Model file for the job. Use its own axes, mm. Face numbers are marked on the shaded views. A direction names the side the tool comes from. Round coordinates to 2 decimals unless told otherwise and drop trailing zeros. Loops run counter-clockwise (first coordinate to the right, second up) from the corner with the lowest first, then second, coordinate; pieces in that order, holes last. Notation, with made-up numbers: M 43.5,50 L 102.5,50 A12 ccw 102.5,59 Z; hole C 52,-7 d1. An arc over 180 degrees is marked long. Use a Markdown table: item, result. Add a question column.
Q1. Probe line 1 (Z direction, x = -33, y = 18) (3 decimals); line 2 (Z direction, x = -33.85, y = 18) (3 decimals); line 3 (X direction, y = 7, z = 7). List the from-to ranges inside material, lowest first. Write a range as from..to.
Q2. Cut at C-C (x = -15.5). Give the cut face in (y, z) (3 decimals).
Q3. Tool access for the marked faces 1, 2, 3 and 4: list every direction of +Z, -Z, +X, -X, +Y, -Y with a clear straight run to the whole face (end or side of a thin tool).
Q4. Pin check, flat tips, straight feed: pin 1 (1.6 mm diameter, centred on x = -36.5, y = 18, fed in from +Z); pin 2 (2.5 mm diameter, centred on x = 5.5, y = 24, fed in from +Z) (3 decimals); pin 3 (6 mm diameter, centred on x = 27, z = -13, fed in from -Y); pin 4 (6 mm diameter, centred on x = -28, z = -6.5, fed in from +Y). Stop position of each tip, or through.
Q5. Cut at A-A (y = 0). Give the cut face in (x, z) (3 decimals).
Q6. Cut at B-B (x = -3). Give the cut face in (y, z) (3 decimals).
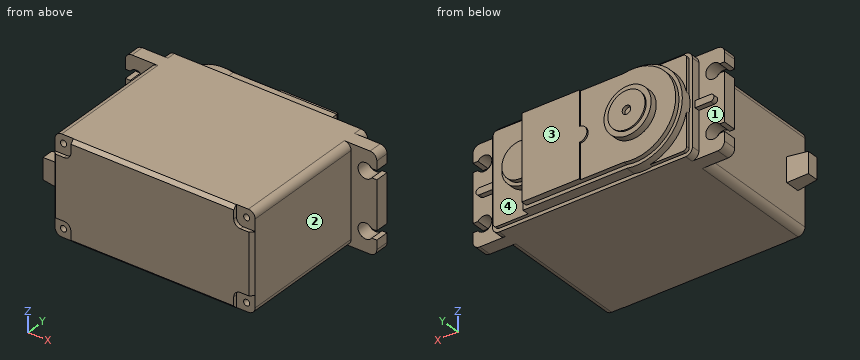
from build123d import *

# Parameters (mm, degrees)
CROQUIS1_W                      = 59.1
CROQUIS1_H                      = 28.85
SALIENTE_EXTRUIR1_DEPTH         = 22.65
CORTAR_EXTRUIR1_DEPTH           = 1.1
CHAFL_N1_SIZE                   = 1
REDONDEO1_R                     = 2
SALIENTE_EXTRUIR2_DEPTH         = 4
REDONDEO2_R                     = 2
SALIENTE_EXTRUIR3_DEPTH         = 1.5
SALIENTE_EXTRUIR4_DEPTH         = 1
SALIENTE_EXTRUIR5_DEPTH         = 3
SALIENTE_EXTRUIR6_DEPTH         = 1.3
CROQUIS8_R                      = 6.96
SALIENTE_EXTRUIR7_DEPTH         = 2
CROQUIS9_R                      = 5.485
SALIENTE_EXTRUIR8_DEPTH         = 0.44
CROQUIS10_R                     = 1.25
CORTAR_EXTRUIR2_DEPTH           = 1
TALADRO_DE_MARGEN_PARA_81_D     = 4.4958
TALADRO_DE_MARGEN_PARA_81_DEPTH = 4
SALIENTE_EXTRUIR9_DEPTH         = 0.5
CROQUIS17_W                     = 7.24
CROQUIS17_H                     = 4.41
CROQUIS18_W                     = 6.24
CROQUIS18_H                     = 3.41


with BuildPart() as part:
    # Croquis1 → Saliente-Extruir1 (new body, symmetric)
    with BuildSketch(Plane(origin=(0, 0, 0), x_dir=(1, 0, 0), z_dir=(0, 1, 0))):
        Rectangle(CROQUIS1_W, CROQUIS1_H)
    extrude(amount=SALIENTE_EXTRUIR1_DEPTH, both=True)

    # Croquis2 → Cortar-Extruir1 (cut)
    with BuildSketch(Plane.XZ.offset(22.65)):
        with BuildLine():
            Line((29.55, 14.425), (24.05, 14.425))
            Line((24.05, 14.425), (24.05, 10.925))
            ThreePointArc((24.05, 10.925), (24.635786438, 9.510786438), (26.05, 8.925))
            Line((26.05, 8.925), (29.55, 8.925))
            Line((29.55, 8.925), (29.55, 14.425))
        make_face()
        with BuildLine():
            Line((-29.55, 14.425), (-29.55, 8.925))
            Line((-29.55, 8.925), (-26.05, 8.925))
            ThreePointArc((-26.05, 8.925), (-24.635786438, 9.510786438), (-24.05, 10.925))
            Line((-24.05, 10.925), (-24.05, 14.425))
            Line((-24.05, 14.425), (-29.55, 14.425))
        make_face()
        with BuildLine():
            Line((24.05, -14.425), (24.05, -10.925))
            ThreePointArc((24.05, -10.925), (24.635786438, -9.510786438), (26.05, -8.925))
            Line((26.05, -8.925), (29.55, -8.925))
            Line((29.55, -8.925), (29.55, -14.425))
            Line((29.55, -14.425), (24.05, -14.425))
        make_face()
        with BuildLine():
            Line((-24.05, -14.425), (-24.05, -10.925))
            ThreePointArc((-24.05, -10.925), (-24.635786438, -9.510786438), (-26.05, -8.925))
            Line((-26.05, -8.925), (-29.55, -8.925))
            Line((-29.55, -8.925), (-29.55, -14.425))
            Line((-29.55, -14.425), (-24.05, -14.425))
        make_face()
    extrude(amount=-CORTAR_EXTRUIR1_DEPTH, mode=Mode.SUBTRACT)

    # Chaflán1
    chafl_n1_edges = [part.edges().sort_by_distance(p)[0] for p in [
        (29.55, -22.65, 0),
        (0, -22.65, 14.425),
        (0, -22.65, -14.425),
        (-29.55, -22.65, 0),
    ]]
    chamfer(chafl_n1_edges, length=CHAFL_N1_SIZE)

    # Redondeo1
    redondeo1_edges = [part.edges().sort_by_distance(p)[0] for p in [
        (29.55, 0.55, 14.425),
        (-29.55, 0.55, 14.425),
        (-29.55, 0.55, -14.425),
        (29.55, 0.55, -14.425),
    ]]
    fillet(redondeo1_edges, radius=REDONDEO1_R)

    # Croquis3 → Saliente-Extruir2 (add)
    with BuildSketch(Plane(origin=(0, 16.15, 0), x_dir=(1, 0, 0), z_dir=(0, 1, 0))):
        with BuildLine():
            Line((27.55, 14.425), (37.15, 14.425))
            Line((37.15, 14.425), (37.15, 9.725))
            Line((37.15, 9.725), (35.599971428, 9.725))
            Line((35.599971428, 9.725), (35.599971428, 7.125))
            Line((35.599971428, 7.125), (37.15, 7.125))
            Line((37.15, 7.125), (37.15, -7.125))
            Line((37.15, -7.125), (35.599971428, -7.125))
            Line((35.599971428, -7.125), (35.599971428, -9.725))
            Line((35.599971428, -9.725), (37.15, -9.725))
            Line((37.15, -9.725), (37.15, -14.425))
            Line((37.15, -14.425), (27.55, -14.425))
            ThreePointArc((27.55, -14.425), (28.964213562, -13.839213562), (29.55, -12.425))
            Line((29.55, -12.425), (29.55, 12.425))
            ThreePointArc((29.55, 12.425), (28.964213562, 13.839213562), (27.55, 14.425))
        make_face()
        with BuildLine():
            Line((-37.15, -9.725), (-37.15, -14.425))
            Line((-37.15, -14.425), (-27.55, -14.425))
            ThreePointArc((-27.55, -14.425), (-28.964213562, -13.839213562), (-29.55, -12.425))
            Line((-29.55, -12.425), (-29.55, 12.425))
            ThreePointArc((-29.55, 12.425), (-28.964213562, 13.839213562), (-27.55, 14.425))
            Line((-27.55, 14.425), (-37.15, 14.425))
            Line((-37.15, 14.425), (-37.15, 9.725))
            Line((-37.15, 9.725), (-35.599971428, 9.725))
            Line((-35.599971428, 9.725), (-35.599971428, 7.125))
            Line((-35.599971428, 7.125), (-37.15, 7.125))
            Line((-37.15, 7.125), (-37.15, -7.125))
            Line((-37.15, -7.125), (-35.599971428, -7.125))
            Line((-35.599971428, -7.125), (-35.599971428, -9.725))
            Line((-35.599971428, -9.725), (-37.15, -9.725))
        make_face()
    extrude(amount=SALIENTE_EXTRUIR2_DEPTH)

    # Redondeo2
    redondeo2_edges = [part.edges().sort_by_distance(p)[0] for p in [
        (37.15, 18.15, 14.425),
        (37.15, 18.15, -14.425),
        (-37.15, 18.15, 14.425),
        (-37.15, 18.15, -14.425),
    ]]
    fillet(redondeo2_edges, radius=REDONDEO2_R)

    # Croquis4 → Saliente-Extruir3 (add)
    with BuildSketch(Plane(origin=(0, 20.15, 0), x_dir=(1, 0, 0), z_dir=(0, 1, 0))):
        with BuildLine():
            Line((34.13221447, -1), (29.55, -1))
            Line((29.55, -1), (29.55, 1))
            Line((29.55, 1), (34.13221447, 1))
            ThreePointArc((34.13221447, 1), (35.13221447, 0), (34.13221447, -1))
        make_face()
        with BuildLine():
            Line((-29.55, -1), (-29.55, 1))
            Line((-29.55, 1), (-34.13221447, 1))
            ThreePointArc((-34.13221447, 1), (-35.13221447, 0), (-34.13221447, -1))
            Line((-34.13221447, -1), (-29.55, -1))
        make_face()
    extrude(amount=SALIENTE_EXTRUIR3_DEPTH)

    # Croquis5 → Saliente-Extruir4 (add)
    with BuildSketch(Plane(origin=(0, 22.65, 0), x_dir=(1, 0, 0), z_dir=(0, 1, 0))):
        with BuildLine():
            Line((-27.55, -13.425), (27.55, -13.425))
            ThreePointArc((27.55, -13.425), (28.257106781, -13.132106781), (28.55, -12.425))
            Line((28.55, -12.425), (28.55, 12.425))
            ThreePointArc((28.55, 12.425), (28.257106781, 13.132106781), (27.55, 13.425))
            Line((27.55, 13.425), (-27.55, 13.425))
            ThreePointArc((-27.55, 13.425), (-28.257106781, 13.132106781), (-28.55, 12.425))
            Line((-28.55, 12.425), (-28.55, -12.425))
            ThreePointArc((-28.55, -12.425), (-28.257106781, -13.132106781), (-27.55, -13.425))
        make_face()
    extrude(amount=SALIENTE_EXTRUIR4_DEPTH)

    # Croquis6 → Saliente-Extruir5 (add)
    with BuildSketch(Plane(origin=(0, 22.65, 0), x_dir=(1, 0, 0), z_dir=(0, 1, 0))):
        with BuildLine():
            Line((-12.39381436, 13.425), (18.25, 13.425))
            Line((18.25, 13.425), (18.25, 6.275))
            ThreePointArc((18.25, 6.275), (24.525, 0), (18.25, -6.275))
            Line((18.25, -6.275), (18.25, -13.425))
            Line((18.25, -13.425), (-12.39381436, -13.425))
            ThreePointArc((-12.39381436, -13.425), (-28.825, 0), (-12.39381436, 13.425))
        make_face()
    extrude(amount=SALIENTE_EXTRUIR5_DEPTH)

    # Croquis7 → Saliente-Extruir6 (add)
    with BuildSketch(Plane(origin=(0, 25.65, 0), x_dir=(1, 0, 0), z_dir=(0, 1, 0))):
        with BuildLine():
            Line((17.25, 5.179346001), (17.25, 12.425))
            Line((17.25, 12.425), (-12.496430998, 12.425))
            ThreePointArc((-12.496430998, 12.425), (-27.825, 0), (-12.496430998, -12.425))
            Line((-12.496430998, -12.425), (17.25, -12.425))
            Line((17.25, -12.425), (17.25, -5.179346001))
            ThreePointArc((17.25, -5.179346001), (23.525, 0), (17.25, 5.179346001))
        make_face()
    extrude(amount=SALIENTE_EXTRUIR6_DEPTH)

    # Croquis8 → Saliente-Extruir7 (add)
    with BuildSketch(Plane(origin=(0, 26.95, 0), x_dir=(1, 0, 0), z_dir=(0, 1, 0))):
        with Locations((-15.125, 0)):
            Circle(CROQUIS8_R)
    extrude(amount=SALIENTE_EXTRUIR7_DEPTH)

    # Croquis9 → Saliente-Extruir8 (add)
    with BuildSketch(Plane(origin=(0, 28.95, 0), x_dir=(1, 0, 0), z_dir=(0, 1, 0))):
        with Locations((-15.125, 0)):
            Circle(CROQUIS9_R)
    extrude(amount=SALIENTE_EXTRUIR8_DEPTH)

    # Croquis10 → Cortar-Extruir2 (cut)
    with BuildSketch(Plane(origin=(0, 29.39, 0), x_dir=(1, 0, 0), z_dir=(0, 1, 0))):
        with Locations((-15.125, 0)):
            Circle(CROQUIS10_R)
    extrude(amount=-CORTAR_EXTRUIR2_DEPTH, mode=Mode.SUBTRACT)

    # Croquis11 → Taladro de margen para M1.61 (revolve, cut)
    with BuildSketch(Plane(origin=(27.05, -21.55, -11.925), x_dir=(0, 0, -1), z_dir=(1, 0, 0))):
        Polygon((0, 0), (0, 5.540774557), (0.9, 5), (0.9, 0), align=None)
    taladro_de_margen_para_m1_61 = revolve(axis=Axis((27.05, -27.9, -11.925), (0, 1, 0)), mode=Mode.SUBTRACT)

    # Simetría1: Taladro de margen para M1.61 across plane
    add(taladro_de_margen_para_m1_61.mirror(Plane.XY), mode=Mode.SUBTRACT)

    # Simetría2: Taladro de margen para M1.61 across plane
    add(taladro_de_margen_para_m1_61.mirror(Plane(origin=(0, 0, 0), x_dir=(0, 0, 1), z_dir=(1, 0, 0))), mode=Mode.SUBTRACT)

    # Simetría2 copy 1 sketch → Simetría2 copy 1 (revolve, cut)
    with BuildSketch(Plane(origin=(-27.05, -21.55, 11.925), x_dir=(0, 0, 1), z_dir=(-1, 0, 0))):
        Polygon((0, 0), (0, 5.540774557), (0.9, 5), (0.9, 0), align=None)
    revolve(axis=Axis((-27.05, -27.9, 11.925), (0, 1, 0)), mode=Mode.SUBTRACT)

    # Taladro de margen para #81
    with Locations(Plane(origin=(0, 20.15, 0), x_dir=(1, 0, 0), z_dir=(0, 1, 0))):
        with Locations((33.85, 8.425), (33.85, -8.425), (-33.85, 8.425), (-33.85, -8.425)):
            Hole(TALADRO_DE_MARGEN_PARA_81_D / 2, depth=TALADRO_DE_MARGEN_PARA_81_DEPTH)

    # Croquis15 → Saliente-Extruir9 (add)
    with BuildSketch(Plane(origin=(0, 26.95, 0), x_dir=(1, 0, 0), z_dir=(0, 1, 0))):
        with BuildLine():
            Line((17.25, 12.425), (0.25, 12.425))
            Line((0.25, 12.425), (0.25, 2.23))
            ThreePointArc((0.25, 2.23), (-1.98, 0), (0.25, -2.23))
            Line((0.25, -2.23), (0.25, -12.425))
            Line((0.25, -12.425), (17.25, -12.425))
            Line((17.25, -12.425), (17.25, 12.425))
        make_face()
    extrude(amount=SALIENTE_EXTRUIR9_DEPTH)

    # Croquis17 → Recubrir1 section 0
    with BuildSketch(Plane.ZY.offset(29.55)):
        with Locations((0, -16.595)):
            Rectangle(CROQUIS17_W, CROQUIS17_H)
    # Croquis18 → Recubrir1 section 1
    with BuildSketch(Plane.ZY.offset(35.55)):
        with Locations((0, -16.595)):
            Rectangle(CROQUIS18_W, CROQUIS18_H)
    loft()


solid = part.part
Checked values:
| question | item | result |
|---|---|---|
| 1 | line 1 | z = -14.425..-10.506, -6.344..6.344, 10.506..14.425 |
| 1 | line 2 | z = -14.425..-10.673, -6.177..6.177, 10.673..14.425 |
| 1 | line 3 | x = -29.55..29.55 |
| 2 | outline | M -22.65,-13.425 L -21.65,-14.425 L 22.65,-14.425 L 22.65,-13.695 L 25.65,-13.695 L 25.65,-12.694 L 26.95,-12.694 L 26.95,-6.95 L 28.95,-6.95 L 28.95,-5.472 L 29.39,-5.472 L 29.39,-1.192 L 28.39,-1.192 L 28.39,1.192 L 29.39,1.192 L 29.39,5.472 L 28.95,5.472 L 28.95,6.95 L 26.95,6.95 L 26.95,12.694 L 25.65,12.694 L 25.65,13.695 L 22.65,13.695 L 22.65,14.425 L -21.65,14.425 L -22.65,13.425 Z |
| 3 | face 1 | -X, +Y |
| 3 | face 2 | +Z, -Z, +X, -Y |
| 3 | face 3 | +Z, -Z, +X, +Y |
| 3 | face 4 | +X, +Y |
| 4 | pin 1 | stops at z = 14.35 |
| 4 | pin 2 | stops at z = 13.425 |
| 4 | pin 3 | stops at y = -22.65 |
| 4 | pin 4 | stops at y = 26.95 |
| 5 | outline | M -29.55,-12.425 A2 ccw -27.55,-14.425 L 27.55,-14.425 A2 ccw 29.55,-12.425 L 29.55,12.425 A2 ccw 27.55,14.425 L -27.55,14.425 A2 ccw -29.55,12.425 Z |
| 6 | outline | M -22.65,-13.425 L -21.65,-14.425 L 22.65,-14.425 L 22.65,-13.425 L 25.65,-13.425 L 25.65,-12.425 L 26.95,-12.425 L 26.95,12.425 L 25.65,12.425 L 25.65,13.425 L 22.65,13.425 L 22.65,14.425 L -21.65,14.425 L -22.65,13.425 Z |
